```python
from build123d import *

# Parameters (mm, degrees)
BOSS_EXTRUDE1_DEPTH = 20
SKETCH4_R           = 7.5
CUT_EXTRUDE1_DEPTH  = 71


with BuildPart() as part:
    # Sketch1 → Boss-Extrude1 (new body)
    with BuildSketch(Plane.XY):
        Polygon((0, 0), (30, 0), (30, 60), (0, 60), (0, 45), (15, 45), (15, 40), (0, 40), (0, 30), (15, 30), (15, 25), (0, 25), (0, 15), (15, 15), (15, 10), (0, 10), align=None)
    extrude(amount=BOSS_EXTRUDE1_DEPTH)

    # Sketch4 → Cut-Extrude1 (cut, through all)
    with BuildSketch(Plane(origin=(0, 60, 0), x_dir=(1, 0, 0), z_dir=(0, 1, 0))):
        with Locations(Location((15, -10, 0), (0, 0, 270))):
            Circle(SKETCH4_R)
    extrude(amount=-CUT_EXTRUDE1_DEPTH, mode=Mode.SUBTRACT)


solid = part.part
```
The listing builds one solid part. Answer for the finished solid, in the listing's coordinates (mm). A direction names the side the tool comes from. Coordinates: 2 decimals unless noted, no trailing zeros. Write each loop counter-clockwise with the first axis right and the second up, starting at its lowest first coordinate (ties: lowest second). Pieces come first, ordered by that corner, then holes.
Q1. The mould has two halves that part along Y. Classify faces 1 (the cylindrical face through (22.436, 30.42, 9.024)), 2 (the flat face through (19, 60, 3)), 3 (the flat face through (6, 15, 10)): released by +Y, released by -Y, zero draft, split by the parting line, or undercut.
Returned:
face 1: zero draft
face 2: released by +Y
face 3: undercut
Q2. Find the intervals of material crossed by line 1 along Z through (x, y) = (15, 35); line 2 along X through (y, z) = (21.5, 10); line 3 along Z through (x, y) = (8.25, 16), in increasing order.
Returned:
line 1: z = 0 to 2.5, 17.5 to 20
line 2: x = 0 to 7.5, 22.5 to 30
line 3: z = 0 to 6.73, 13.27 to 20
Q3. Section C-C, the plane y = 24 is taken. Write down the section's boundary in (x, z).
Returned:
outline: (0, 0) - (30, 0) - (30, 20) - (0, 20) - close; hole circle Ø15 at (15, 10)
Q4. Given P1, Ø2, axis at y = 27.5, z = 1, coming from the -X side, flat-ended and moving along its own axis, determine where the tip first touches the part or whether it passes through.
Returned:
P1: stops at x = 15
Q5. Which of the six approach directions +Z, -Z, +X, -X, +Y, -Y give full straight-line access (tool end or side, diameter ignored) to faces 4 (the flat face through (11, 0, 3)), 5 (the flat face through (15, 28, 19))?
Returned:
face 4: +Z, -Z, +X, -X, -Y
face 5: +Z, -Z, -X
Q6. Section B-B, the plane z = 10 is taken. Write down the section's boundary in (x, y), then the cut area to 4 significant figures.
Returned:
outline: (0, 0) - (7.5, 0) - (7.5, 10) - (0, 10) - close; (0, 15) - (7.5, 15) - (7.5, 25) - (0, 25) - close; (0, 30) - (7.5, 30) - (7.5, 40) - (0, 40) - close; (0, 45) - (7.5, 45) - (7.5, 60) - (0, 60) - close; (22.5, 0) - (30, 0) - (30, 60) - (22.5, 60) - close
area: 787.5 mm2
Q7. Section D-D, the plane z = 1.5 is taken. Write down the section's boundary in (x, y), then the cut area to 4 significant figures.
Returned:
outline: (0, 0) - (30, 0) - (30, 60) - (0, 60) - (0, 45) - (15, 45) - (15, 40) - (0, 40) - (0, 30) - (15, 30) - (15, 25) - (0, 25) - (0, 15) - (15, 15) - (15, 10) - (0, 10) - close
area: 1,575 mm2
Q8. Section A-A, the plane x = 19.5 is taken. Write down the section's boundary in (y, z), then the cut area to 3 significant figures.
Returned:
outline: (0, 0) - (60, 0) - (60, 4) - (0, 4) - close; (0, 16) - (60, 16) - (60, 20) - (0, 20) - close
area: 480 mm2
